Check sheet for the modelled part. Datum: model origin and axes. Units: mm. A direction names the side the tool comes from. Coordinates: 2 decimals unless noted, no trailing zeros. Loops run counter-clockwise (first coordinate to the right, second up) from the corner with the lowest first, then second, coordinate; pieces in that order, holes last. Notation, with made-up numbers: (-1, -26) - (18, -26) arc R30 ccw to (18, 12) - close; hole circle Ø1 at (83.5, 18). An arc over 180 degrees is marked (long way). Write each question's results on one line, items separated by ' | '. Start each with the question number.
1. Draft check along Z on faces 1 (the face through (0, -3, 11.43)), 2 (the face through (13.97, -8, 10)), 3 (the face through (-11.47, -12.68, -11.43)). Enter one of: released by +Z, released by -Z, zero draft, split by the parting line, or undercut.
2. Cross-section at C-C (z = -1). Record the cut outline in (x, y) (3 decimals), and give its area (3 significant figures).
3. Cross-section at D-D (y = 5.5). Record the cut outline in (x, z), and give its area (3 significant figures).
4. Cross-section at A-A (y = -8.5). Record the cut outline in (x, z) (3 decimals).
5. Tool access check on faces 4 (the face through (-16, -5.08, -10)), 5 (the face through (12.01, -12.68, 9.72)), 6 (the face through (24, 10, -2.286)), 7 (the face through (8.89, -8, -10)). Record the directions out of +Z, -Z, +X, -X, +Y, -Y that give a thin tool (end or side, any length) a straight path to the whole face; none if there is none.
6. Cross-section at B-B (x = -2). Record the cut outline in (y, z) (3 decimals), and give its area (3 significant figures).
7. Thickness scan on line 1 (Z direction, x = 10.5, y = -5.25) (3 decimals); line 2 (Y direction, x = -16, z = 2.25); line 3 (Z direction, x = 14.5, y = 3.25). Record the ranges inside material, lowest first. Write a range as [from, to].
8. Gauge pin test, flat ends, axial feed: P1, Ø1, axis at y = -7, z = -10, coming from the -X side; P2, Ø2, axis at x = -10.5, z = 11, coming from the -Y side; P3, Ø1, axis at x = 13.5, z = 8, coming from the +Y side; P4, Ø2, axis at x = 13.5, z = -10, coming from the -Y side. Record the tip position at first contact, or that the pin passes through.
```python
from build123d import *

# Parameters (mm, degrees)
BOSS_EXTRUDE1_DEPTH = 19.05
SKETCH2_W           = 4.572
SKETCH2_H           = 1.952455346
BOSS_EXTRUDE2_DEPTH = 9.525
SKETCH3_R           = 0.976227673
BOSS_EXTRUDE3_DEPTH = 4.572
SKETCH4_R           = 0.381
CUT_EXTRUDE1_DEPTH  = 35.526057015
SKETCH5_W           = 5.08
SKETCH5_H           = 6.35
SKETCH5_W_2         = 17.78
CUT_EXTRUDE2_DEPTH  = 40.070443522
SKETCH6_R           = 0.9525
BOSS_EXTRUDE4_DEPTH = 2.54


with BuildPart() as part:
    # Sketch1 → Boss-Extrude1 (new, symmetric)
    with BuildSketch(Plane(origin=(0, 0, 0), x_dir=(0, 0, -1), z_dir=(1, 0, 0))):
        with BuildLine():
            Line((-9.525, 0), (-9.525, -11.43))
            Line((-9.525, -11.43), (-11.43, -11.43))
            Line((-11.43, -11.43), (-11.43, 0))
            ThreePointArc((-11.43, 0), (0, 11.43), (11.43, 0))
            Line((11.43, 0), (11.43, -11.43))
            Line((11.43, -11.43), (9.525, -11.43))
            Line((9.525, -11.43), (9.525, 0))
            ThreePointArc((9.525, 0), (0, 9.525), (-9.525, 0))
        make_face()
    extrude(amount=BOSS_EXTRUDE1_DEPTH, both=True)

    # Sketch2 → Boss-Extrude2 (add, symmetric)
    with BuildSketch(Plane(origin=(19.05, 0, 0), x_dir=(0, 0, -1), z_dir=(1, 0, 0))):
        with Locations((0, 10.222839431)):
            Rectangle(SKETCH2_W, SKETCH2_H)
    extrude(amount=BOSS_EXTRUDE2_DEPTH, both=True)

    # Sketch3 → Boss-Extrude3 (add)
    with BuildSketch(Plane(origin=(0, 0, -2.286), x_dir=(-1, 0, 0), z_dir=(0, 0, -1))):
        with Locations((-28.575, 10.222839431)):
            Circle(SKETCH3_R)
    extrude(amount=-BOSS_EXTRUDE3_DEPTH)

    # Sketch4 → Cut-Extrude1 (cut, through all)
    with BuildSketch(Plane(origin=(0, 0, -2.286), x_dir=(-1, 0, 0), z_dir=(0, 0, -1))):
        with Locations((-28.575, 10.222839431)):
            Circle(SKETCH4_R)
    extrude(amount=-CUT_EXTRUDE1_DEPTH, mode=Mode.SUBTRACT)

    # Sketch5 → Cut-Extrude2 (cut, through all)
    with BuildSketch(Plane(origin=(0, 0, -11.43), x_dir=(-1, 0, 0), z_dir=(0, 0, -1))):
        with Locations((-16.51, -8.255)):
            Rectangle(SKETCH5_W, SKETCH5_H)
        with Locations((0, -8.255)):
            Rectangle(SKETCH5_W_2, SKETCH5_H)
        with Locations((16.51, -8.255)):
            Rectangle(SKETCH5_W, SKETCH5_H)
    extrude(amount=-CUT_EXTRUDE2_DEPTH, mode=Mode.SUBTRACT)

    # Sketch6 → Boss-Extrude4 (add)
    with BuildSketch(Plane.XZ.offset(11.43)):
        with Locations(Location((11.43, -10.4775, 0), (0, 0, 270))):
            Circle(SKETCH6_R)
        with Locations(Location((11.43, 10.4775, 0), (0, 0, 90))):
            Circle(SKETCH6_R)
        with Locations(Location((-11.43, 10.4775, 0), (0, 0, 270))):
            Circle(SKETCH6_R)
        with Locations(Location((-11.43, -10.4775, 0), (0, 0, 90))):
            Circle(SKETCH6_R)
    extrude(amount=BOSS_EXTRUDE4_DEPTH)


solid = part.part
```
Established:
1) face 1: released by +Z | face 2: zero draft | face 3: undercut
2) outline: (-19.05, 9.472) - (9.525, 9.472) - (9.525, 9.247) - (28.575, 9.247) arc R0.976 ccw to (28.575, 11.199) - (19.05, 11.199) - (19.05, 11.386) - (-19.05, 11.386) - close; hole circle Ø0.762 at (28.575, 10.223) | area: 94.7 mm^2
3) outline: (-19.05, -10.02) - (19.05, -10.02) - (19.05, -7.78) - (-19.05, -7.78) - close; (-19.05, 7.78) - (19.05, 7.78) - (19.05, 10.02) - (-19.05, 10.02) - close | area: 171 mm^2
4) outline: (-13.97, -11.43) - (-8.89, -11.43) - (-8.89, -9.525) - (-13.97, -9.525) - close; (-13.97, 9.525) - (-8.89, 9.525) - (-8.89, 11.43) - (-13.97, 11.43) - close; (8.89, -11.43) - (13.97, -11.43) - (13.97, -9.525) - (8.89, -9.525) - close; (8.89, 9.525) - (13.97, 9.525) - (13.97, 11.43) - (8.89, 11.43) - close
5) face 4: +Z, -Z, -X, -Y | face 5: -Y | face 6: -Z, +X, +Y, -Y | face 7: +Z, -Z, -Y
6) outline: (-5.08, -11.43) - (0, -11.43) arc R11.43 ccw to (0, 11.43) - (-5.08, 11.43) - (-5.08, 9.525) - (0, 9.525) arc R9.525 cw to (0, -9.525) - (-5.08, -9.525) - close | area: 82.1 mm^2
7) line 1: [-11.43, -9.525], [9.525, 11.43] | line 2: [9.26, 11.21] | line 3: [-10.96, -8.95], [8.95, 10.96]
8) P1: x = -13.97 | P2: y = -13.97 | P3: y = 8.63 | P4: y = -11.43
